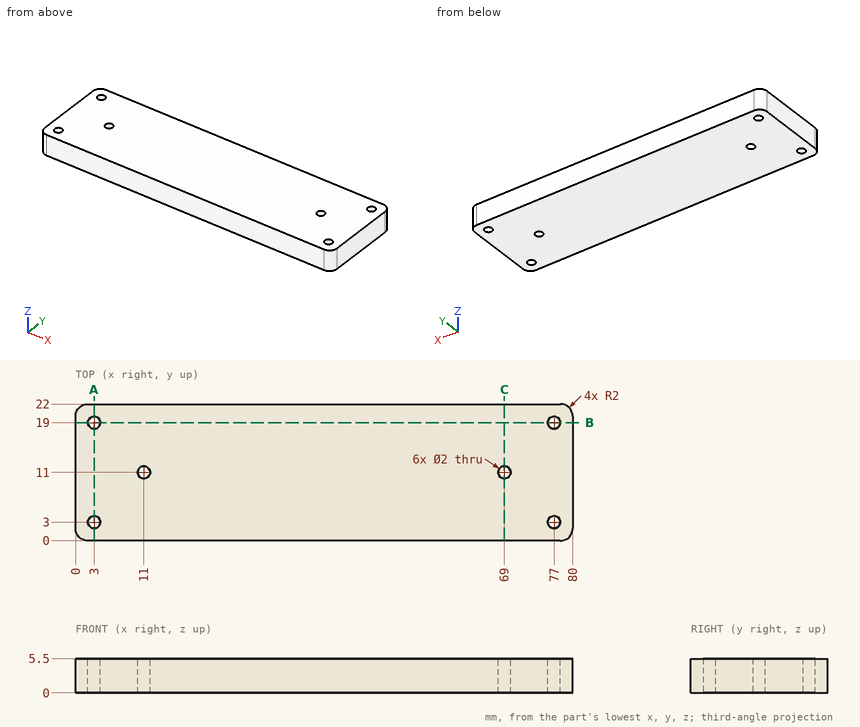
Geometry check sheet. Reference: drawing and pictorial views, mm from the part's lowest x, y, z. Round coordinates to 2 decimals unless told otherwise and drop trailing zeros. Write each loop counter-clockwise with the first axis right and the second up, starting at its lowest first coordinate (ties: lowest second). Pieces come first, ordered by that corner, then holes. Notation, with made-up numbers: (57, -6) -> (96, -6) arc R22 cw to (96, 12) -> close; hole circle Ø6 at (67, 35.5). An arc over 180 degrees is marked (long way). Put each result on its own line as item: value.
1) Cross-section at B-B, the plane y = 19. Enter the section's corners in (x, z).
Recorded:
outline: (0, 0) -> (2, 0) -> (2, 5.5) -> (0, 5.5) -> close; (4, 0) -> (76, 0) -> (76, 5.5) -> (4, 5.5) -> close; (78, 0) -> (80, 0) -> (80, 5.5) -> (78, 5.5) -> close
2) Thickness scan on probe 1 along X at (y, z) = (11, 2.9); probe 2 along X at (y, z) = (3, 4.15); probe 3 along Y at (x, z) = (69, 2.8). Record the ranges inside material, lowest first. Write a range as from..to.
Recorded:
probe 1: x = 0..10, 12..68, 70..80
probe 2: x = 0..2, 4..76, 78..80
probe 3: y = 0..10, 12..22
3) Cross-section at C-C, the plane x = 69. Enter the section's corners in (y, z), plus the area to 3 significant figures.
Recorded:
outline: (0, 0) -> (10, 0) -> (10, 5.5) -> (0, 5.5) -> close; (12, 0) -> (22, 0) -> (22, 5.5) -> (12, 5.5) -> close
area: 110 mm2
4) Cross-section at A-A, the plane x = 3. Enter the section's corners in (y, z).
Recorded:
outline: (0, 0) -> (2, 0) -> (2, 5.5) -> (0, 5.5) -> close; (4, 0) -> (18, 0) -> (18, 5.5) -> (4, 5.5) -> close; (20, 0) -> (22, 0) -> (22, 5.5) -> (20, 5.5) -> close
5) Depth check by flat-ended pin: P1, Ø1.2, axis at x = 11, y = 11, coming from the +Z side. Enter the tip coordinate at first touch or a pass-through.
Recorded:
P1: passes through
